The listing builds one solid part. Answer for the finished solid, in the listing's coordinates (mm). A direction names the side the tool comes from. Round coordinates to 2 decimals unless told otherwise and drop trailing zeros. Write each loop counter-clockwise with the first axis right and the second up, starting at its lowest first coordinate (ties: lowest second). Pieces come first, ordered by that corner, then holes.
Item 1: Find section C-C on x = -65. Give the vertices of the cut face in (y, z).
Item 2: Find section B-B on z = 3.5. Give the vertices of the cut face in (x, y).
Item 3: A tool of negligible diameter and unlimited length cuts with its end or side. For faces 1 (the face through (52.093, 10, 11)), 2 (the face through (-1, 30, 11)), from which of +Z, -Z, +X, -X, +Y, -Y can it reach the whole face along a straight path? Write none if from no direction.
Item 4: For a pull along Z with two mould halves and no side action, classify faces 3 (the face through (1, 22, 20)), 4 (the face through (1, 24, 0)), 5 (the face through (-52.093, 10, 11)) as +Z half, -Z half, draft (parallel to the pull), parting line (faces both ways), or undercut.
Item 5: Find section A-A on y = 15. Give the vertices of the cut face in (x, z), then the cut area to 3 significant figures.
Item 6: Each of these flat-tipped pins is pushed along its axis until it touches: pin 1 (4.5 mm diameter, centred on x = 65, y = 5, fed in from -Z); pin 2 (5.5 mm diameter, centred on x = -18.5, z = 13.5, fed in from -Y). Where does it stop, or does it pass through?
Item 7: Find the intervals of material crossed by probe 1 along X at (y, z) = (5, 9.75); probe 2 along X at (y, z) = (15, 3.75); probe 3 along X at (y, z) = (5.5, 5.5), in increasing order.
Item 8: Find section D-D on y = 5. Give the vertices of the cut face in (x, z), then the cut area to 3 significant figures.
```python
from build123d import *

# Parameters (mm, degrees)
F1_DEPTH     = 20
F3_D         = 5
F5_T1_DEPTH  = 150
F5_T3_DEPTH  = 40
F5_T5_DEPTH  = 27.906979831
F5_T7_DEPTH  = 25
F5_T9_DEPTH  = 104.186040338
F5_T11_DEPTH = 27.906979831
F5_T21_DEPTH = 30
F5_T25_DEPTH = 109.186040338
F5_T32_DEPTH = 109.186040338
F5_T36_DEPTH = 30


# Not quite as in the source:
# - a fillet or chamfer that OpenCascade refuses, or shapes differently, is made with other operations: its cross-section is extruded or revolved along the edge and cut away or added


with BuildPart() as f1:
    # F0 (on Top) → F1 (new body)
    with BuildSketch(Plane.XY):
        Polygon((70, 30), (0, 30), (0, 20), (52.093020169, 20), (52.093020169, 0), (70, 0), align=None)
    extrude(amount=F1_DEPTH)

    # F3 (through all)
    with Locations(Plane.XY.offset(20)):
        with Locations((65, 5)):
            Hole(F3_D / 2)

    # F4: F1 across face


with BuildPart() as f1_1:
    add(f1.part)
    add(f1.part.mirror(Plane(origin=(0, 25, 10), x_dir=(0, -1, 0), z_dir=(-1, 0, 0))))

    # F5: fillet of radius 2 on 10 edges, made by hand

    # F5_s2 → F5_t1 (cut)
    with BuildSketch(Plane.YZ.offset(-75)):
        with BuildLine():
            ThreePointArc((30, 2), (29.4142135624, 0.5857864376), (28, 0))
            Line((28, 0), (30, 0))
            Line((30, 0), (30, 2))
        make_face()
    extrude(amount=F5_T1_DEPTH, mode=Mode.SUBTRACT)

    # F5_s4 → F5_t3 (cut)
    with BuildSketch(Plane.XZ.offset(-35)):
        with BuildLine():
            ThreePointArc((-68, 0), (-69.4142135624, 0.5857864376), (-70, 2))
            Line((-70, 2), (-70, 0))
            Line((-70, 0), (-68, 0))
        make_face()
        with BuildLine():
            ThreePointArc((68, 0), (69.4142135624, 0.5857864376), (70, 2))
            Line((70, 2), (70, 0))
            Line((70, 0), (68, 0))
        make_face()
    extrude(amount=F5_T3_DEPTH, mode=Mode.SUBTRACT)

    # F5_s6 → F5_t5 (cut)
    with BuildSketch(Plane.YZ.offset(-75)):
        with BuildLine():
            ThreePointArc((2, 0), (0.5857864376, 0.5857864376), (0, 2))
            Line((0, 2), (0, 0))
            Line((0, 0), (2, 0))
        make_face()
    extrude(amount=F5_T5_DEPTH, mode=Mode.SUBTRACT)

    # F5_s8 → F5_t7 (cut)
    with BuildSketch(Plane.XZ.offset(-20)):
        with BuildLine():
            ThreePointArc((-54.093020169, 0), (-52.6788066067, 0.5857864376), (-52.093020169, 2))
            Line((-52.093020169, 2), (-52.093020169, 0))
            Line((-52.093020169, 0), (-54.093020169, 0))
        make_face()
        with BuildLine():
            ThreePointArc((54.093020169, 0), (52.6788066067, 0.5857864376), (52.093020169, 2))
            Line((52.093020169, 2), (52.093020169, 0))
            Line((52.093020169, 0), (54.093020169, 0))
        make_face()
    extrude(amount=F5_T7_DEPTH, mode=Mode.SUBTRACT)

    # F5_s10 → F5_t9 (cut)
    with BuildSketch(Plane.YZ.offset(-52.093020169)):
        with BuildLine():
            ThreePointArc((22, 0), (20.5857864376, 0.5857864376), (20, 2))
            Line((20, 2), (20, 0))
            Line((20, 0), (22, 0))
        make_face()
    extrude(amount=F5_T9_DEPTH, mode=Mode.SUBTRACT)

    # F5_s12 → F5_t11 (cut)
    with BuildSketch(Plane.YZ.offset(47.093020169)):
        with BuildLine():
            ThreePointArc((2, 0), (0.5857864376, 0.5857864376), (0, 2))
            Line((0, 2), (0, 0))
            Line((0, 0), (2, 0))
        make_face()
    extrude(amount=F5_T11_DEPTH, mode=Mode.SUBTRACT)

    # F5_s13 → F5_t14 (revolve, cut)
    with BuildSketch(Plane.XZ.offset(-5)):
        with BuildLine():
            ThreePointArc((69.5, 0), (68.0857864376, 0.5857864376), (67.5, 2))
            Line((67.5, 2), (67.5, 0))
            Line((67.5, 0), (69.5, 0))
        make_face()
    revolve(axis=Axis((65, 5, 0), (0, 0, 1)), mode=Mode.SUBTRACT)

    # F5_s15 → F5_t16 (revolve, cut)
    with BuildSketch(Plane.XZ.offset(-5)):
        with BuildLine():
            ThreePointArc((-69.5, 0), (-68.0857864376, 0.5857864376), (-67.5, 2))
            Line((-67.5, 2), (-67.5, 0))
            Line((-67.5, 0), (-69.5, 0))
        make_face()
    revolve(axis=Axis((-65, 5, 0), (0, 0, -1)), mode=Mode.SUBTRACT)


with BuildPart() as f5_tool19:
    # F5_s20 → F5_t21 (new body)
    with BuildSketch(Plane.XZ.offset(-25)):
        with BuildLine():
            ThreePointArc((-54.093020169, 0), (-52.6788066067, 0.5857864376), (-52.093020169, 2))
            Line((-52.093020169, 2), (-52.093020169, 0))
            Line((-52.093020169, 0), (-54.093020169, 0))
        make_face()
    extrude(amount=F5_T21_DEPTH)

    split(bisect_by=Plane.XZ.offset(-20), keep=Keep.BOTTOM)


with BuildPart() as f5_tool23:
    # F5_s24 → F5_t25 (new body)
    with BuildSketch(Plane.YZ.offset(52.093020169)):
        with BuildLine():
            ThreePointArc((22, 0), (20.5857864376, 0.5857864376), (20, 2))
            Line((20, 2), (20, 0))
            Line((20, 0), (22, 0))
        make_face()
    extrude(amount=-F5_T25_DEPTH)

    split(bisect_by=Plane.YZ.offset(-52.093020169), keep=Keep.BOTTOM)


with BuildPart() as f5_tool19_1:
    add(f5_tool19.part)

    # F5_t27: intersect F5_tool23
    add(f5_tool23.part, mode=Mode.INTERSECT)


with BuildPart() as f1_2:
    add(f1_1.part)

    # F5_t17: cut F5_tool19
    add(f5_tool19_1.part, mode=Mode.SUBTRACT)


with BuildPart() as f5_tool30:
    # F5_s31 → F5_t32 (new body)
    with BuildSketch(Plane.YZ.offset(57.093020169)):
        with BuildLine():
            ThreePointArc((22, 0), (20.5857864376, 0.5857864376), (20, 2))
            Line((20, 2), (20, 0))
            Line((20, 0), (22, 0))
        make_face()
    extrude(amount=-F5_T32_DEPTH)

    split(bisect_by=Plane.YZ.offset(52.093020169), keep=Keep.TOP)


with BuildPart() as f5_tool34:
    # F5_s35 → F5_t36 (new body)
    with BuildSketch(Plane.XZ.offset(-25)):
        with BuildLine():
            ThreePointArc((54.093020169, 0), (52.6788066067, 0.5857864376), (52.093020169, 2))
            Line((52.093020169, 2), (52.093020169, 0))
            Line((52.093020169, 0), (54.093020169, 0))
        make_face()
    extrude(amount=F5_T36_DEPTH)

    split(bisect_by=Plane.XZ.offset(-20), keep=Keep.BOTTOM)


with BuildPart() as f5_tool30_1:
    add(f5_tool30.part)

    # F5_t38: intersect F5_tool34
    add(f5_tool34.part, mode=Mode.INTERSECT)


with BuildPart() as f1_3:
    add(f1_2.part)

    # F5_t28: cut F5_tool30
    add(f5_tool30_1.part, mode=Mode.SUBTRACT)


solid = f1_3.part
```
Check values:
1. outline: (0, 2) arc R2 ccw to (1.25, 0.15) arc R2 ccw to (2.5, 2) - (2.5, 20) - (0, 20) - close; (7.5, 2) arc R2 ccw to (9.5, 0) - (28, 0) arc R2 ccw to (30, 2) - (30, 20) - (7.5, 20) - close
2. outline: (-70, 0) - (-52.09, 0) - (-52.09, 20) - (52.09, 20) - (52.09, 0) - (70, 0) - (70, 30) - (-70, 30) - close; hole circle Ø5 at (-65, 5); hole circle Ø5 at (65, 5)
3. face 1: +Z, -Z, -Y
3. face 2: +Z, -Z, +X, -X, +Y
4. face 3: +Z half
4. face 4: -Z half
4. face 5: draft
5. outline: (-70, 2) arc R2 ccw to (-68, 0) - (-54.09, 0) arc R2 ccw to (-52.09, 2) - (-52.09, 20) - (-70, 20) - close; (52.09, 2) arc R2 ccw to (54.09, 0) - (68, 0) arc R2 ccw to (70, 2) - (70, 20) - (52.09, 20) - close
5. area: 713 mm2
6. pin 1: passes through
6. pin 2: stops at y = 20
7. probe 1: x = -70 to -67.5, -62.5 to -52.09, 52.09 to 62.5, 67.5 to 70
7. probe 2: x = -70 to -52.09, 52.09 to 70
7. probe 3: x = -70 to -67.45, -62.55 to -52.09, 52.09 to 62.55, 67.45 to 70
8. outline: (-70, 2) arc R2 ccw to (-68.75, 0.15) arc R2 ccw to (-67.5, 2) - (-67.5, 20) - (-70, 20) - close; (-62.5, 2) arc R2 ccw to (-60.5, 0) - (-54.09, 0) arc R2 ccw to (-52.09, 2) - (-52.09, 20) - (-62.5, 20) - close; (52.09, 2) arc R2 ccw to (54.09, 0) - (60.5, 0) arc R2 ccw to (62.5, 2) - (62.5, 20) - (52.09, 20) - close; (67.5, 2) arc R2 ccw to (68.75, 0.15) arc R2 ccw to (70, 2) - (70, 20) - (67.5, 20) - close
8. area: 510 mm2
